```python
from build123d import *

# Parameters (mm, degrees)
ESQUISSE1_R             = 5
BOSS_EXTRU_1_DEPTH      = 50
ENL_V_MAT_EXTRU_2_DEPTH = 48


with BuildPart() as part:
    # Esquisse1 → Boss.-Extru.1 (new body)
    with BuildSketch(Plane.XY):
        with BuildLine():
            Line((-15, -17.5), (15, -17.5))
            Line((15, -17.5), (15, 17.5))
            ThreePointArc((15, 17.5), (0, 32.5), (-15, 17.5))
            Line((-15, 17.5), (-15, -17.5))
        make_face()
        with Locations((0, 17.5)):
            Circle(ESQUISSE1_R, mode=Mode.SUBTRACT)
    extrude(amount=-BOSS_EXTRU_1_DEPTH)

    # Esquisse2 → Enlèv. mat.-Extru.2 (cut)
    with BuildSketch(Plane(origin=(0, 0, -50), x_dir=(-1, 0, 0), z_dir=(0, 0, -1))):
        with BuildLine():
            Line((-13, 17.5), (-13, -15.5))
            Line((-13, -15.5), (13, -15.5))
            Line((13, -15.5), (13, 17.5))
            ThreePointArc((13, 17.5), (0, 30.5), (-13, 17.5))
        make_face()
    extrude(amount=-ENL_V_MAT_EXTRU_2_DEPTH, mode=Mode.SUBTRACT)


solid = part.part
```
Geometry: final body of the model. Coordinates: model frame, mm. A direction names the side the tool comes from. Round coordinates to 2 decimals unless told otherwise and drop trailing zeros. Order: outer loops, then holes, each group sorted by start corner. A loop starts at its lowest first (then second) coordinate and runs counter-clockwise, first axis right, second up. Notation, with made-up numbers: (-27.75, 50.5) -> (-14.75, 50.5) arc R26 ccw to (-14.75, 68.5) -> close; hole circle Ø11 at (76, 43.5). An arc over 180 degrees is marked (long way). Use one line per item in the form item = value.
(1) Section B-B on z = -9. Return loops of the section in (x, y), and give its area (3 significant figures).
Results list:
outline = (-15, -17.5) -> (15, -17.5) -> (15, 17.5) arc R15 ccw to (-15, 17.5) -> close; hole (-13, -15.5) -> (13, -15.5) -> (13, 17.5) arc R13 ccw to (-13, 17.5) -> close
area = 280 mm^2
(2) Draft query along Y for faces 1 (the face through (-13, 1, -26)), 2 (the face through (0, -17.5, -25)), 3 (the face through (-15, 0, -25)), 4 (the face through (-1.08, 12.62, -0.99)). Return one class per face: pulls with the +Y half, pulls with the -Y half, needs draft (parallel to the pull), parting line crosses it, or undercut.
Results list:
face_1 = undercut
face_2 = pulls with the -Y half
face_3 = needs draft
face_4 = undercut
(3) Ray query, probe 1 along X at (y, z) = (17, -30.5); probe 2 along X at (y, z) = (17, -1); probe 3 along Y at (x, z) = (-2, -35). Return the intervals inside material, ascending. Write a range as [from, to].
Results list:
probe_1 = [-15, -13], [13, 15]
probe_2 = [-15, -4.97], [4.97, 15]
probe_3 = [-17.5, -15.5], [30.35, 32.37]
(4) Access query for faces 5 (the face through (0, 8, 0)), 6 (the face through (0, 8, -2)). Directions: +Z, -Z, +X, -X, +Y, -Y. A direction counts if a zero-diameter tool reaches every point of the face in a straight line with its end or side. Return the directions, or none.
Results list:
face_5 = +Z, +X, -X, +Y, -Y
face_6 = -Z
(5) First-contact query: pin 1 Ø12 at (x, y) = (5, -8.5) entering from -Z; pin 2 Ø8 at (x, z) = (4.5, -20.5) entering from +Y. Flat tips, straight axial feed; report the tip coordinate or a pass-through.
Results list:
pin_1 = -2
pin_2 = 32.49
(6) Section D-D on x = 6.75. Return loops of the section in (y, z).
Results list:
outline = (-17.5, -50) -> (-15.5, -50) -> (-15.5, -2) -> (28.61, -2) -> (28.61, -50) -> (30.9, -50) -> (30.9, 0) -> (-17.5, 0) -> close
(7) Section C-C on y = -0.5. Return loops of the section in (x, z).
Results list:
outline = (-15, -50) -> (-13, -50) -> (-13, -2) -> (13, -2) -> (13, -50) -> (15, -50) -> (15, 0) -> (-15, 0) -> close
(8) Section A-A on x = 0. Return loops of the section in (y, z).
Results list:
outline = (-17.5, -50) -> (-15.5, -50) -> (-15.5, -2) -> (12.5, -2) -> (12.5, 0) -> (-17.5, 0) -> close; (22.5, -2) -> (30.5, -2) -> (30.5, -50) -> (32.5, -50) -> (32.5, 0) -> (22.5, 0) -> close
